Can you work these out from the model? Positions are in its coordinate system, mm. A direction names the side the tool comes from. Round coordinates to 2 decimals unless told otherwise and drop trailing zeros. Loops run counter-clockwise (first coordinate to the right, second up) from the corner with the lowest first, then second, coordinate; pieces in that order, holes last.
from build123d import *

# Parameters (mm, degrees)
CYLINDER294_R     = 54.5
CYLINDER294_DEPTH = 28
CYLINDER289_R     = 1.5
CYLINDER289_DEPTH = 20
CYLINDER290_R     = 1.5
CYLINDER290_DEPTH = 20
CYLINDER291_R     = 1.5
CYLINDER291_DEPTH = 20
CYLINDER292_R     = 1.5
CYLINDER292_DEPTH = 20
CYLINDER293_R     = 1.5
CYLINDER293_DEPTH = 20
CYLINDER288_R     = 1.5
CYLINDER288_DEPTH = 20
CYLINDER299_R     = 3
CYLINDER299_DEPTH = 3
CYLINDER298_R     = 3
CYLINDER298_DEPTH = 3
CYLINDER297_R     = 3
CYLINDER297_DEPTH = 3
CYLINDER296_R     = 3
CYLINDER296_DEPTH = 3
CYLINDER295_R     = 3
CYLINDER295_DEPTH = 3
CYLINDER300_R     = 3
CYLINDER300_DEPTH = 3
BOX133_W          = 10
BOX133_H          = 108
BOX133_DEPTH      = 45


with BuildPart() as obj1:
    # Cylinder294 → Cylinder294 (new body)
    with BuildSketch(Plane.XY.offset(9)):
        Circle(CYLINDER294_R)
    extrude(amount=CYLINDER294_DEPTH)


with BuildPart() as obj2:
    # Cylinder289 → Cylinder289 (new body)
    with BuildSketch(Plane(origin=(45, -19, -5), x_dir=(0, 0, -1), z_dir=(1, 0, 0))):
        Circle(CYLINDER289_R)
    extrude(amount=CYLINDER289_DEPTH)


with BuildPart() as obj3:
    # Cylinder290 → Cylinder290 (new body)
    with BuildSketch(Plane(origin=(45, 51, 7), x_dir=(0, 0, -1), z_dir=(1, 0, 0))):
        Circle(CYLINDER290_R)
    extrude(amount=CYLINDER290_DEPTH)


with BuildPart() as obj4:
    # Cylinder291 → Cylinder291 (new body)
    with BuildSketch(Plane(origin=(45, -51, 7), x_dir=(0, 0, -1), z_dir=(1, 0, 0))):
        Circle(CYLINDER291_R)
    extrude(amount=CYLINDER291_DEPTH)


with BuildPart() as obj5:
    # Cylinder292 → Cylinder292 (new body)
    with BuildSketch(Plane(origin=(45, -51, 30), x_dir=(0, 0, -1), z_dir=(1, 0, 0))):
        Circle(CYLINDER292_R)
    extrude(amount=CYLINDER292_DEPTH)


with BuildPart() as obj6:
    # Cylinder293 → Cylinder293 (new body)
    with BuildSketch(Plane(origin=(45, 51, 30), x_dir=(0, 0, -1), z_dir=(1, 0, 0))):
        Circle(CYLINDER293_R)
    extrude(amount=CYLINDER293_DEPTH)


with BuildPart() as compound582:
    # Cylinder288 → Cylinder288 (new body)
    with BuildSketch(Plane(origin=(45, 19, -5), x_dir=(0, 0, -1), z_dir=(1, 0, 0))):
        Circle(CYLINDER288_R)
    extrude(amount=CYLINDER288_DEPTH)

    # Compound582: union obj2, obj3, obj4, obj5, obj6
    add(obj2.part)
    add(obj3.part)
    add(obj4.part)
    add(obj5.part)
    add(obj6.part)


with BuildPart() as obj7:
    # Cylinder299 → Cylinder299 (new body)
    with BuildSketch(Plane(origin=(53, -19, -5), x_dir=(0, 0, -1), z_dir=(1, 0, 0))):
        Circle(CYLINDER299_R)
    extrude(amount=CYLINDER299_DEPTH)


with BuildPart() as obj8:
    # Cylinder298 → Cylinder298 (new body)
    with BuildSketch(Plane(origin=(53, 51, 7), x_dir=(0, 0, -1), z_dir=(1, 0, 0))):
        Circle(CYLINDER298_R)
    extrude(amount=CYLINDER298_DEPTH)


with BuildPart() as obj9:
    # Cylinder297 → Cylinder297 (new body)
    with BuildSketch(Plane(origin=(53, -51, 7), x_dir=(0, 0, -1), z_dir=(1, 0, 0))):
        Circle(CYLINDER297_R)
    extrude(amount=CYLINDER297_DEPTH)


with BuildPart() as obj10:
    # Cylinder296 → Cylinder296 (new body)
    with BuildSketch(Plane(origin=(53, -51, 30), x_dir=(0, 0, -1), z_dir=(1, 0, 0))):
        Circle(CYLINDER296_R)
    extrude(amount=CYLINDER296_DEPTH)


with BuildPart() as obj11:
    # Cylinder295 → Cylinder295 (new body)
    with BuildSketch(Plane(origin=(53, 51, 30), x_dir=(0, 0, -1), z_dir=(1, 0, 0))):
        Circle(CYLINDER295_R)
    extrude(amount=CYLINDER295_DEPTH)


with BuildPart() as compound583:
    # Cylinder300 → Cylinder300 (new body)
    with BuildSketch(Plane(origin=(53, 19, -5), x_dir=(0, 0, -1), z_dir=(1, 0, 0))):
        Circle(CYLINDER300_R)
    extrude(amount=CYLINDER300_DEPTH)

    # Compound583: union obj7, obj8, obj9, obj10, obj11
    add(obj7.part)
    add(obj8.part)
    add(obj9.part)
    add(obj10.part)
    add(obj11.part)


with BuildPart() as cut359:
    # Box133 → Box133 (new body)
    with BuildSketch(Plane(origin=(46, -54, -8), x_dir=(1, 0, 0), z_dir=(0, 0, 1))):
        with Locations((5, 54)):
            Rectangle(BOX133_W, BOX133_H)
    extrude(amount=BOX133_DEPTH)

    # Cut358: cut Compound583
    add(compound583.part, mode=Mode.SUBTRACT)

    # Cut360: cut Compound582
    add(compound582.part, mode=Mode.SUBTRACT)

    # Cut359: cut obj1
    add(obj1.part, mode=Mode.SUBTRACT)


solid = cut359.part
(1) For faces 1 (the flat face through (53, -52.3, 5.7)), 2 (the flat face through (49, 0, 9)), 3 (the flat face through (56, -1, 14)), which set-ups out of +Z, -Z, +X, -X, +Y, -Y let a thin tool reach every point of the face, with its end or its side?
Worked answers:
face 1: +X
face 2: +Z, -X
face 3: +Z, -Z, +X, +Y, -Y
(2) If we section it at D-D, the plane z = 18: List the corners of the cut face in (x, y) for me.
Worked answers:
outline: (46, -54) - (56, -54) - (56, 54) - (46, 54) - (46, 29.23) arc R54.5 cw to (46, -29.23) - close
(3) If I drill on line 1 (Z direction, x = 50, y = 51); line 2 (Y direction, x = 50, z = -5); line 3 (Z direction, x = 53.95, y = 51), over which ranges is the centre line in solid material (lowest first)?
Worked answers:
line 1: z = -8 to 5.5, 8.5 to 28.5, 31.5 to 37
line 2: y = -54 to -20.5, -17.5 to 17.5, 20.5 to 54
line 3: z = -8 to 4, 10 to 27, 33 to 37
(4) If we mould it in two halves opening along Z, with no side actions, what happens to faces 4 (the flat face through (51, 54, 14)), 5 (the cylindrical face through (54.48, -21.93, -4.35)), 6 (the flat face through (51, 1, -8)), 7 (the cylindrical face through (49.451, -52.464, 7.325))? For each: released by +Z, released by -Z, zero draft, split by the parting line, or undercut.
Worked answers:
face 4: zero draft
face 5: undercut
face 6: released by -Z
face 7: undercut
(5) If we section it at B-B, the plane x = 49: List the corners of the cut face in (y, z) for me.
Worked answers:
outline: (-54, -8) - (54, -8) - (54, 37) - (23.86, 37) - (23.86, 9) - (-23.86, 9) - (-23.86, 37) - (-54, 37) - close; hole circle Ø3 at (-51, 7); hole circle Ø3 at (-51, 30); hole circle Ø3 at (-19, -5); hole circle Ø3 at (19, -5); hole circle Ø3 at (51, 7); hole circle Ø3 at (51, 30)
(6) Will these pins go through, and if not, where does the flat tip stop? P1, Ø7, axis at y = 19, z = -5, coming from the +X side; P2, Ø3, axis at y = -51, z = 6, coming from the +X side; P3, Ø2.5, axis at y = 19, z = -5, coming from the +X side; P4, Ø2, axis at y = 17.5, z = 17, coming from the -X side.
Worked answers:
P1: stops at x = 56
P2: stops at x = 53
P3: passes through
P4: stops at x = 51.26
(7) If we section it at A-A, the plane z = -5: List the corners of the cut face in (x, y) for me, then the cut area to 3 significant figures.
Worked answers:
outline: (46, -54) - (56, -54) - (56, -22) - (53, -22) - (53, -20.5) - (46, -20.5) - close; (46, -17.5) - (53, -17.5) - (53, -16) - (56, -16) - (56, 16) - (53, 16) - (53, 17.5) - (46, 17.5) - close; (46, 20.5) - (53, 20.5) - (53, 22) - (56, 22) - (56, 54) - (46, 54) - close
area: 1,000 mm2
(8) If we section it at C-C, the plane y = 0: List the corners of the cut face in (x, z) for me.
Worked answers:
outline: (46, -8) - (56, -8) - (56, 37) - (54.5, 37) - (54.5, 9) - (46, 9) - close
